The model under review builds one solid part; all positions refer to its coordinate system, in mm. A direction names the side the tool comes from. Round coordinates to 2 decimals unless told otherwise and drop trailing zeros. Write each loop counter-clockwise with the first axis right and the second up, starting at its lowest first coordinate (ties: lowest second). Pieces come first, ordered by that corner, then holes. Notation, with made-up numbers: (-19.5, -12.5) - (26.5, -12.5) arc R32 ccw to (26.5, 19.5) - close; hole circle Ø8 at (9.5, -16). An arc over 180 degrees is marked (long way). One line per question, with ' | ' between items. Start each with the question number.
```python
from build123d import *

# Parameters (mm, degrees)
F1_DEPTH = 63.5
F0_W     = 25.4
F0_H     = 28.575
F2_DEPTH = 25.4
F3_DEPTH = 7.9375
F5_R     = 6.35


with BuildPart() as f1:
    # F0 (on Front) → F1 (new body, symmetric)
    with BuildSketch(Plane.XZ):
        Polygon((22.225, 9.525), (-41.275, 9.525), (-41.275, -9.525), (41.275, -9.525), (41.275, 9.525), align=None)
    extrude(amount=F1_DEPTH, both=True)

    # F0 (on Front) → F2 (join, symmetric)
    with BuildSketch(Plane.XZ):
        with BuildLine():
            Line((22.225, 27.0002), (22.225, 9.525))
            Line((22.225, 9.525), (41.275, 9.525))
            Line((41.275, 9.525), (41.275, 27.0002))
            ThreePointArc((41.275, 27.0002), (45.92468, 38.22552), (57.15, 42.8752))
            Line((57.15, 42.8752), (60.325, 42.8752))
            Line((60.325, 42.8752), (60.325, 55.5752))
            Line((60.325, 55.5752), (60.325, 61.9252))
            Line((60.325, 61.9252), (57.15, 61.9252))
            add(Edge.make_bspline(
                [(53.755209, 61.759818), (54.878671, 61.824514), (56.010282, 61.879666), (57.15, 61.9252)],
                knots=[108.887606, 108.887606, 108.887606, 108.887606, 111.504536, 111.504536, 111.504536, 111.504536], degree=3))
            ThreePointArc((53.755209, 61.759818), (31.281885, 50.464988), (22.225, 27.0002))
        make_face()
        Polygon((60.325, 66.675), (60.325, 61.9252), (60.325, 55.5752), (60.325, 42.8752), (60.325, 38.1), (85.725, 38.1), (85.725, 66.675), align=None)
        with Locations((98.425, 52.3875)):
            Rectangle(F0_W, F0_H)
    extrude(amount=F2_DEPTH, both=True)

    # F0 (on Front) → F3 (join, symmetric)
    with BuildSketch(Plane.XZ):
        with BuildLine():
            add(Edge.make_bspline(
                [(-41.275, 9.525), (-25.63058, 39.853167), (7.009152, 59.067885), (53.755209, 61.759818)],
                knots=[0, 0, 0, 0, 108.887606, 108.887606, 108.887606, 108.887606], degree=3))
            Line((-41.275, 9.525), (22.225, 9.525))
            Line((22.225, 9.525), (22.225, 27.0002))
            ThreePointArc((22.225, 27.0002), (31.281885, 50.464988), (53.755209, 61.759818))
        make_face()
    extrude(amount=F3_DEPTH, both=True)

    # F0 (on Front) → F4 (revolve)
    with BuildSketch(Plane.XZ):
        with Locations((98.425, 52.3875)):
            Rectangle(F0_W, F0_H)
    revolve(axis=Axis((85.725, 0, 52.3875), (0, 0, -1)))

    # F5
    f5_edges = [f1.edges().sort_by_distance(p)[0] for p in [
        (41.275, -63.5, 0),
        (41.275, 63.5, 0),
        (-41.275, -63.5, 0),
        (-41.275, 63.5, 0),
    ]]
    fillet(f5_edges, radius=F5_R)


solid = f1.part
```
1. Add section C-C, the plane x = 70. Write out the cut boundary in (y, z) (3 decimals).
2. Clearance check with flat-ended pins moving along their axes: P1, Ø18.5, axis at y = -12.5, z = 12, coming from the +X side (3 decimals); P2, Ø5.5, axis at y = -1, z = 40, coming from the -X side; P3, Ø8.5, axis at y = -18.5, z = 19.5, coming from the -X side (3 decimals). State where each tip first meets the part, or that it passes through.
3. The part is to be moulded in two halves that separate along X. For faces 6 (the face through (-4, 7.938, 30)), 7 (the face through (60.325, 0, 41)), 8 (the face through (-39.365, -61.689, -0.133)), say which applies: pulls with the +X half, pulls with the -X half, needs draft (parallel to the pull), parting line crosses it, or undercut.
4. Add section B-B, the plane y = 45.5. Write out the cut boundary in (x, z) (3 decimals), then the cut area to 3 significant figures.
5. Add section A-A, the plane z = 6.5. Write out the cut boundary in (x, y) (3 decimals).
6. Wall thickness on line 1 along Y through (x, z) = (-26.5, 10); line 2 along Z through (x, y) = (21, 53) (3 decimals); line 3 along Y through (x, z) = (39, 28): over which ranges is each line inside the solid? List them lowest first. Write a range as [from, to].
7. Machinability: for faces 1 (the face through (-1, -1, -9.525)), 2 (the face through (41.275, -1, 4)), 3 (the face through (66, -25.4, 45)), 4 (the face through (31.525, 16.547, 50.731)), 5 (the face through (22.225, -17, 18)), which of the approach directions +Z, -Z, +X, -X, +Y, -Y give a long, thin tool a straight path to every point of the face, cutting with its end or side? Answer none if there is none.
Geometry check:
1) outline: (-25.4, 38.1) - (25.4, 38.1) - (25.4, 66.675) - (-25.4, 66.675) - close
2) P1: stops at x = 41.275 | P2: stops at x = -18.48 | P3: stops at x = 22.225
3) face 6: needs draft | face 7: undercut | face 8: pulls with the -X half
4) outline: (-41.275, -9.525) - (41.275, -9.525) - (41.275, 9.525) - (-41.275, 9.525) - close | area: 1,570 mm2
5) outline: (-41.275, -57.15) arc R6.35 ccw to (-34.925, -63.5) - (34.925, -63.5) arc R6.35 ccw to (41.275, -57.15) - (41.275, 57.15) arc R6.35 ccw to (34.925, 63.5) - (-34.925, 63.5) arc R6.35 ccw to (-41.275, 57.15) - close
6) line 1: y = [-7.94, 7.94] | line 2: z = [-9.525, 9.525] | line 3: y = [-25.4, 25.4]
7) face 1: -Z, +X, -X, +Y, -Y | face 2: -Z, +X, +Y, -Y | face 3: +Z, +X, -X, -Y | face 4: +Z, -X, +Y | face 5: +Z, -X, -Y
